Build history of the part. All positions in model axes, mm. Round coordinates to 2 decimals unless told otherwise and drop trailing zeros. Loops run counter-clockwise (first coordinate to the right, second up) from the corner with the lowest first, then second, coordinate; pieces in that order, holes last. Notation, with made-up numbers: (84.5, -6) - (114.5, -6) arc R36 cw to (114.5, 32) - close; hole circle Ø7 at (-11, 81.5). An arc over 180 degrees is marked (long way). Use a Markdown table: item, result.
from build123d import *

# Parameters (mm, degrees)
SKETCH1_R          = 8.35025
BASE_EXTRUDE_DEPTH = 4.7625


with BuildPart() as part:
    # Sketch1 → Base-Extrude (new body)
    with BuildSketch(Plane.XY):
        with BuildLine():
            Line((19.05, 8.599479175), (19.05, -8.599479175))
            ThreePointArc((19.05, -8.599479175), (16.589286609, -22.069863356), (9.525, -33.800260413))
            ThreePointArc((9.525, -33.800260413), (0, -38.1), (-9.525, -33.800260413))
            ThreePointArc((-9.525, -33.800260413), (-16.589286609, -22.069863356), (-19.05, -8.599479175))
            Line((-19.05, -8.599479175), (-19.05, 8.599479175))
            ThreePointArc((-19.05, 8.599479175), (-16.589286609, 22.069863356), (-9.525, 33.800260413))
            ThreePointArc((-9.525, 33.800260413), (0, 38.1), (9.525, 33.800260413))
            ThreePointArc((9.525, 33.800260413), (16.589286609, 22.069863356), (19.05, 8.599479175))
        make_face()
        with Locations(Location((0, 0, 0), (0, 0, 180))):
            Circle(SKETCH1_R, mode=Mode.SUBTRACT)
    extrude(amount=BASE_EXTRUDE_DEPTH)


solid = part.part
Q1. Probe line 1 (X direction, y = -5, z = 2.95); line 2 (Y direction, x = 4, z = 0.3); line 3 (Y direction, x = 0, z = 2.2). List the from-to ranges inside material, lowest first.
Results found:
| item | result |
|---|---|
| line 1 | x = -19.05 to -6.69, 6.69 to 19.05 |
| line 2 | y = -37.45 to -7.33, 7.33 to 37.45 |
| line 3 | y = -38.1 to -8.35, 8.35 to 38.1 |
Q2. Cut at A-A, the plane x = 0. List the corners of the cut face in (y, z), plus the area to 3 significant figures.
Results found:
| item | result |
|---|---|
| outline | (-38.1, 0) - (-8.35, 0) - (-8.35, 4.76) - (-38.1, 4.76) - close; (8.35, 0) - (38.1, 0) - (38.1, 4.76) - (8.35, 4.76) - close |
| area | 283 mm2 |
Q3. Drop flat-ended pins along their axis: pin 1 (2 mm diameter, centred on x = -14.5, z = 3.5, fed in from +Y); pin 2 (5 mm diameter, centred on x = 4, y = 11.5, fed in from -Z); pin 3 (1 mm diameter, centred on x = -1, z = 1, fed in from +Y). Give the stop position or say it passes through.
Results found:
| item | result |
|---|---|
| pin 1 | stops at y = 28.4 |
| pin 2 | stops at z = 0 |
| pin 3 | stops at y = 38.09 |
Q4. Cut at D-D, the plane y = -16.5. List the corners of the cut face in (x, z), plus the area to 3 significant figures.
Results found:
| item | result |
|---|---|
| outline | (-18.22, 0) - (18.22, 0) - (18.22, 4.76) - (-18.22, 4.76) - close |
| area | 174 mm2 |
Q5. Cut at B-B, the plane y = 0. List the corners of the cut face in (x, z).
Results found:
| item | result |
|---|---|
| outline | (-19.05, 0) - (-8.35, 0) - (-8.35, 4.76) - (-19.05, 4.76) - close; (8.35, 0) - (19.05, 0) - (19.05, 4.76) - (8.35, 4.76) - close |
